Geometry: final body of the model. Coordinates: model frame, mm. Give positions to 0.01 mm unless a question says otherwise; leave off trailing zeros. Loops run counter-clockwise (first coordinate to the right, second up) from the corner with the lowest first, then second, coordinate; pieces in that order, holes last. Notation, with made-up numbers: (63.25, -17.75) -> (117.25, -17.75) arc R27 ccw to (117.25, 3.25) -> close; hole circle Ø3 at (80, 42). An arc over 180 degrees is marked (long way). Answer in a Markdown table with one row per item. Add a question column.
1) Line query: line 1 (Z direction, x = 31, y = -1.6); line 2 (Z direction, x = 42.5, y = -0.55); line 3 (X direction, y = -0.85, z = -7.25). Output: solid intervals per line, ascending. Write a range as from..to.
2) Section query C-C (x = 42.5). Return the cut outline in (y, z), plus the area to 3 significant figures.
3) Section query B-B (y = -1.5). Give the number of separate pieces and of enclosed holes in the cut face, plus the area to 3 significant figures.
4) First-contact query: P1, Ø1.8, axis at x = -42.5, z = -6, coming from the +Y side; P2, Ø3.5, axis at x = -42.5, z = 6, coming from the -Y side. Flat tips, straight axial feed; report the tip coordinate or a pass-through.
5) Section query A-A (x = 28.5). Return the cut outline in (y, z).
```python
from build123d import *

# Parameters (mm, degrees)
F0_W     = 84
F0_H     = 21
F0_W_2   = 78
F0_H_2   = 3
F0_W_3   = 72
F0_R     = 1.5
F1_DEPTH = 2
F2_W     = 2
F2_H     = 21
F3_DEPTH = 5
F4_W     = 2
F4_H     = 21
F5_DEPTH = 5
F6_R     = 1.5
F7_DEPTH = 25
F8_R     = 1


with BuildPart() as f1:
    # F0 (on Front) → F1 (new body)
    with BuildSketch(Plane.XZ):
        Rectangle(F0_W, F0_H)
        with Locations((0, -6)):
            Rectangle(F0_W_2, F0_H_2, mode=Mode.SUBTRACT)
        with Locations((-3, 6)):
            Rectangle(F0_W_3, F0_H_2, mode=Mode.SUBTRACT)
        Rectangle(F0_W_2, F0_H_2, mode=Mode.SUBTRACT)
        with Locations((37.5, 6)):
            Circle(F0_R, mode=Mode.SUBTRACT)
    extrude(amount=F1_DEPTH)

    # F2 (on face) → F3 (join)
    with BuildSketch(Plane.YZ.offset(42)):
        with Locations((-1, 0)):
            Rectangle(F2_W, F2_H)
    extrude(amount=F3_DEPTH)

    # F4 (on face) → F5 (join)
    with BuildSketch(Plane(origin=(-42, 0, 0), x_dir=(0, -1, 0), z_dir=(-1, 0, 0))):
        with Locations((1, 0)):
            Rectangle(F4_W, F4_H)
    extrude(amount=F5_DEPTH)

    # F6 (on face) → F7 (cut)
    with BuildSketch(Plane.XZ.offset(2)):
        with Locations((-42.5, 6)):
            Circle(F6_R)
        with Locations((-42.5, -6)):
            Circle(F6_R)
        with Locations((42.5, 6)):
            Circle(F6_R)
        with Locations((42.5, -6)):
            Circle(F6_R)
    extrude(amount=-F7_DEPTH, mode=Mode.SUBTRACT)

    # F8
    f8_edges = [f1.edges().sort_by_distance(p)[0] for p in [
        (-39, -1, 7.5),
        (-39, -1, 1.5),
        (-39, -1, -4.5),
        (-39, -1, 4.5),
        (-39, -1, -1.5),
        (-39, -1, -7.5),
        (33, -1, 7.5),
        (39, -1, 1.5),
        (39, -1, -4.5),
        (39, -1, -7.5),
        (39, -1, -1.5),
        (33, -1, 4.5),
    ]]
    fillet(f8_edges, radius=F8_R)


solid = f1.part
```
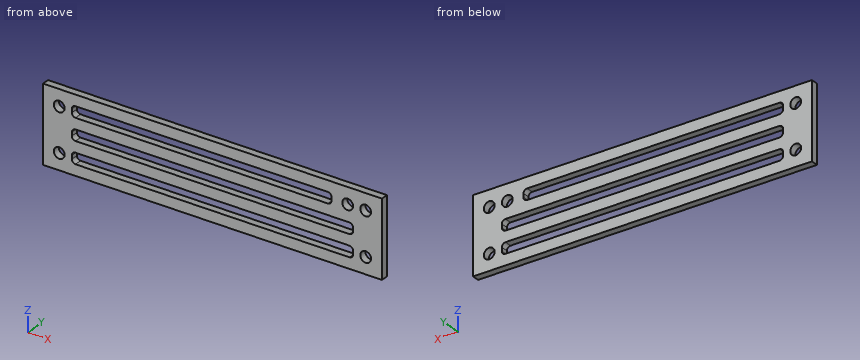
Evaluation:
| question | item | result |
|---|---|---|
| 1 | line 1 | -10.5..-7.5, -4.5..-1.5, 1.5..4.5, 7.5..10.5 |
| 1 | line 2 | -10.5..-7.5, -4.5..4.5, 7.5..10.5 |
| 1 | line 3 | -47..-43.33, -41.67..-38.66, 38.66..41.67, 43.33..47 |
| 2 | outline | (-2, -10.5) -> (0, -10.5) -> (0, -7.5) -> (-2, -7.5) -> close; (-2, -4.5) -> (0, -4.5) -> (0, 4.5) -> (-2, 4.5) -> close; (-2, 7.5) -> (0, 7.5) -> (0, 10.5) -> (-2, 10.5) -> close |
| 2 | area | 30.0 mm² |
| 3 | separate pieces | 1 |
| 3 | enclosed holes | 8 |
| 3 | area | 1,260 mm² |
| 4 | P1 | through |
| 4 | P2 | y = -2 |
| 5 | outline | (-2, -10.5) -> (0, -10.5) -> (0, -7.5) -> (-2, -7.5) -> close; (-2, -4.5) -> (0, -4.5) -> (0, -1.5) -> (-2, -1.5) -> close; (-2, 1.5) -> (0, 1.5) -> (0, 4.5) -> (-2, 4.5) -> close; (-2, 7.5) -> (0, 7.5) -> (0, 10.5) -> (-2, 10.5) -> close |
